```python
from build123d import *

# Parameters (mm, degrees)
F0_W     = 800
F0_H     = 1100
F1_DEPTH = 800
F4_W     = 300
F4_H     = 300
F5_DEPTH = 200


with BuildPart() as f1:
    # F0 (on Front) → F1 (new body)
    with BuildSketch(Plane.XZ):
        with Locations((0, 650)):
            Rectangle(F0_W, F0_H)
    extrude(amount=F1_DEPTH)

    # F2 (on face) → F3 (revolve)
    with BuildSketch(Plane.XY.offset(1200)):
        with BuildLine():
            ThreePointArc((300, -400), (0, -100), (-300, -400))
            Line((-300, -400), (300, -400))
        make_face()
    revolve(axis=Axis((0, -400, 1200), (1, 0, 0)))

    # F4 (on face) → F5 (cut)
    with BuildSketch(Plane(origin=(0, 0, 100), x_dir=(1, 0, 0), z_dir=(0, 0, -1))):
        with Locations((-249, 649)):
            Rectangle(F4_W, F4_H)
        with Locations((249, 649)):
            Rectangle(F4_W, F4_H)
        with Locations((249, 151)):
            Rectangle(F4_W, F4_H)
        with Locations((-249, 151)):
            Rectangle(F4_W, F4_H)
    extrude(amount=-F5_DEPTH, mode=Mode.SUBTRACT)


solid = f1.part
```
The listing builds one solid part. Answer for the finished solid, in the listing's coordinates (mm). A direction names the side the tool comes from. Coordinates: 2 decimals unless noted, no trailing zeros. Write each loop counter-clockwise with the first axis right and the second up, starting at its lowest first coordinate (ties: lowest second). Pieces come first, ordered by that corner, then holes. Notation, with made-up numbers: (48, 85.5) - (77, 85.5) arc R10 ccw to (77, 98.5) - close; hole circle Ø3 at (-20, 37). An arc over 180 degrees is marked (long way). Return JSON: item names as keys, results as strings. Group by question number.
Q1. Flat-ended cylindrical pins translate along their axes: pin 1 Ø12 at (x, y) = (-88, -616) entering from +Z; pin 2 Ø4 at (x, y) = (-144, -124) entering from -Z; pin 3 Ø1.5 at (x, y) = (209.5, -362) entering from +Z. Find the tip coordinate at first contact, or state that the pin passes through.
Q2. The part is cut by section C-C on x = 201.5. Write down the section's boundary in (y, z).
Q3. The part is cut by section B-B on y = -751. Write down the section's boundary in (x, z).
Q4. For a pull along X with two mould halves and no side action, classify faces 1 (the flat face through (-6, -800, 658)), 2 (the flat face through (-251, -1, 199)), 3 (the flat face through (-400, -394, 642)), 4 (the flat face through (247, -651, 300)) as +X half, -X half, draft (parallel to the pull), parting line (faces both ways), or undercut.
Q5. The part is cut by section A-A on z = 265. Write down the section's boundary in (x, y).
Q6. Which of the six approach directions +Z, -Z, +X, -X, +Y, -Y give full straight-line access (tool end or side, diameter ignored) to faces 5 (the flat face through (-6, -394, 100)), 6 (the flat face through (-99, -149, 199)), 7 (the flat face through (172, -661, 1200))?
Q7. Find the intervals of material crossed by line 1 along Z through (x, y) = (218, -37.5); line 2 along Z through (x, y) = (-144, -331.5); line 3 along Y through (x, z) = (-148, 1323), in increasing order. Write a range as [from, to].
Q8. The part is cut by section D-D on x = -126. Write down the section's boundary in (y, z), and give its area (3 significant figures).
Evaluation:
{
 "1": {"pin 1": "stops at z = 1395.86", "pin 2": "stops at z = 300", "pin 3": "stops at z = 1412.1"},
 "2": {"outline": "(-800, 100) - (-799, 100) - (-799, 300) - (-499, 300) - (-499, 100) - (-301, 100) - (-301, 300) - (-1, 300) - (-1, 100) - (0, 100) - (0, 1200) - (-177.74, 1200) arc R222.26 ccw to (-622.26, 1200) - (-800, 1200) - close"},
 "3": {"outline": "(-400, 100) - (-399, 100) - (-399, 300) - (-99, 300) - (-99, 100) - (99, 100) - (99, 300) - (399, 300) - (399, 100) - (400, 100) - (400, 1200) - (-400, 1200) - close"},
 "4": {"face 1": "draft", "face 2": "undercut", "face 3": "-X half", "face 4": "undercut"},
 "5": {"outline": "(-400, -800) - (400, -800) - (400, 0) - (-400, 0) - close; hole (-399, -799) - (-99, -799) - (-99, -499) - (-399, -499) - close; hole (-399, -301) - (-99, -301) - (-99, -1) - (-399, -1) - close; hole (99, -799) - (399, -799) - (399, -499) - (99, -499) - close; hole (99, -301) - (399, -301) - (399, -1) - (99, -1) - close"},
 "6": {"face 5": "-Z, +X, -X, +Y, -Y", "face 6": "-Z", "face 7": "+Z"},
 "7": {"line 1": "z = [300, 1200]", "line 2": "z = [100, 1454.11]", "line 3": "y = [-630.15, -169.85]"},
 "8": {"outline": "(-800, 100) - (-799, 100) - (-799, 300) - (-499, 300) - (-499, 100) - (-301, 100) - (-301, 300) - (-1, 300) - (-1, 100) - (0, 100) - (0, 1200) - (-127.74, 1200) arc R272.26 ccw to (-672.26, 1200) - (-800, 1200) - close", "area": "876,000 mm2"}
}
